```python
from build123d import *

# Parameters (mm, degrees)
SKETCH1_W           = 82.55
SKETCH1_H           = 25.4
SKETCH1_R           = 2.921
BOSS_EXTRUDE1_DEPTH = 1.1176
MOVE_FACE2_BY       = 0.09652


with BuildPart() as part:
    # Sketch1 → Boss-Extrude1 (new body)
    with BuildSketch(Plane(origin=(0, 0, 0), x_dir=(1, 0, 0), z_dir=(0, 1, 0))):
        Rectangle(SKETCH1_W, SKETCH1_H)
        with Locations(Location((-34.925, 0, 0), (0, 0, 270))):
            Circle(SKETCH1_R, mode=Mode.SUBTRACT)
        with Locations(Location((34.925, 0, 0), (0, 0, 270))):
            Circle(SKETCH1_R, mode=Mode.SUBTRACT)
    extrude(amount=BOSS_EXTRUDE1_DEPTH)

    # Move Face2: a face moved outward by 0.09652
    extrude(part.faces().sort_by_distance((0, 1.1176, 0))[0], amount=MOVE_FACE2_BY, dir=(0, 1, 0))


solid = part.part
```
Can you work these out from the model? Positions are in its coordinate system, mm. Round coordinates to 2 decimals unless told otherwise and drop trailing zeros. Loops run counter-clockwise (first coordinate to the right, second up) from the corner with the lowest first, then second, coordinate; pieces in that order, holes last. Notation, with made-up numbers: M 60,34.25 L 96,34.25 A36 cw 96,73.25 Z; hole C 74,-35 d3. An arc over 180 degrees is marked long. Write item = value, one per line. Start each with the question number.
(1) Suppose I cut it at B-B on x = 34. Write out the boundary of the cut face in (y, z), plus the area to 3 significant figures.
(2) Suppose I cut it at C-C on y = 0.7. Write out the boundary of the cut face in (x, z) (3 decimals).
(3) I'm going to push a flat-ended pin straight in: P1, Ø4.5, axis at x = -34.925, z = 0, coming from the -Y side. Where does the tip first touch, or does it pass through?
(4) Suppose I cut it at A-A on z = 0. Write out the boundary of the cut face in (x, y) (3 decimals), plus the area to 3 significant figures.
(5) I need wall thicknesses on line 1 along X through (y, z) = (0.6, 0) (3 decimals); line 2 along X through (y, z) = (0.35, -1.5) (3 decimals). Which ranges of each line are inside material? Lowest first, please.
(6) If we mould it in two halves opening along Z, with no side actions, what happens to faces 1 (the face through (32.334, 0.599, 1.348)), 2 (the face through (-1, 1.214, 0))? For each: released by +Z, released by -Z, zero draft, split by the parting line, or undercut.
Answer block:
q1.outline = M 0,-12.7 L 1.21,-12.7 L 1.21,-2.77 L 0,-2.77 Z; M 0,2.77 L 1.21,2.77 L 1.21,12.7 L 0,12.7 Z
q1.area = 24.1 mm²
q2.outline = M -41.275,-12.7 L 41.275,-12.7 L 41.275,12.7 L -41.275,12.7 Z; hole C -34.925,0 d5.842; hole C 34.925,0 d5.842
q3.P1 = through
q4.outline = M -41.275,0 L -37.846,0 L -37.846,1.214 L -41.275,1.214 Z; M -32.004,0 L 32.004,0 L 32.004,1.214 L -32.004,1.214 Z; M 37.846,0 L 41.275,0 L 41.275,1.214 L 37.846,1.214 Z
q4.area = 86.0 mm²
q5.line_1 = -41.275 to -37.846, -32.004 to 32.004, 37.846 to 41.275
q5.line_2 = -41.275 to -37.431, -32.419 to 32.419, 37.431 to 41.275
q6.face_1 = undercut
q6.face_2 = zero draft
